```python
from build123d import *

# Parameters (mm, degrees)
SKETCH070_W         = 19.5
SKETCH070_H         = 35
PAD035_DEPTH        = 6
SKETCH074_W         = 15.5
SKETCH074_H         = 31
POCKET025_DEPTH     = 4
SKETCH071_W         = 11.5
SKETCH071_H         = 27
POCKET023_DEPTH     = 2.001
SKETCH069_W         = 11.5
SKETCH069_H         = 4
POCKET024_DEPTH     = 6.001
REVOLUTION007_ANGLE = 180
REVOLUTION008_ANGLE = -180


with BuildPart() as part:
    # Sketch070 → Pad035 (new body)
    with BuildSketch(Plane.XY):
        with Locations((9.75, 17.5)):
            Rectangle(SKETCH070_W, SKETCH070_H)
    extrude(amount=PAD035_DEPTH)

    # Sketch074 (on Face6 of Pad035) → Pocket025 (cut)
    with BuildSketch(Plane.XY.offset(6)):
        with Locations((9.75, 17.5)):
            Rectangle(SKETCH074_W, SKETCH074_H)
    extrude(amount=-POCKET025_DEPTH, mode=Mode.SUBTRACT)

    # Sketch071 (on Face11 of Pocket025) → Pocket023 (cut, through all)
    with BuildSketch(Plane.XY.offset(2)):
        with Locations((9.75, 17.5)):
            Rectangle(SKETCH071_W, SKETCH071_H)
    extrude(amount=-POCKET023_DEPTH, mode=Mode.SUBTRACT)

    # Sketch069 (on Face5 of Pocket023) → Pocket024 (cut, through all)
    with BuildSketch(Plane.XY.offset(6)):
        with Locations((9.75, 2)):
            Rectangle(SKETCH069_W, SKETCH069_H)
    extrude(amount=-POCKET024_DEPTH, mode=Mode.SUBTRACT)

    # Sketch075 (on Face18 of Pocket024) → Revolution007 (revolve)
    with BuildSketch(Plane.YZ.offset(2)):
        with BuildLine():
            ThreePointArc((6.5, 5), (5.5, 6), (4.5, 5))
            Line((4.5, 5), (6.5, 5))
        make_face()
        with BuildLine():
            ThreePointArc((30.5, 5), (29.5, 6), (28.5, 5))
            Line((28.5, 5), (30.5, 5))
        make_face()
    revolve(axis=Axis((2, 6.5, 5), (0, 1, 0)), revolution_arc=REVOLUTION007_ANGLE)

    # Sketch076 (on Face17 of Revolution007) → Revolution008 (revolve)
    with BuildSketch(Plane(origin=(17.5, 0, 0), x_dir=(0, -1, 0), z_dir=(-1, 0, 0))):
        with BuildLine():
            ThreePointArc((-28.5, 5), (-29.5, 6), (-30.5, 5))
            Line((-30.5, 5), (-28.5, 5))
        make_face()
        with BuildLine():
            ThreePointArc((-4.5, 5), (-5.5, 6), (-6.5, 5))
            Line((-6.5, 5), (-4.5, 5))
        make_face()
    revolve(axis=Axis((17.5, 6.5, 5), (0, 1, 0)), revolution_arc=REVOLUTION008_ANGLE)


solid = part.part
```
The model under review builds one solid part; all positions refer to its coordinate system, in mm. A direction names the side the tool comes from. Coordinates: 2 decimals unless noted, no trailing zeros. Write each loop counter-clockwise with the first axis right and the second up, starting at its lowest first coordinate (ties: lowest second). Pieces come first, ordered by that corner, then holes.
1) We need section C-C on x = 13. State the section outline as (y, z) points.
2) Machinability: for faces 1 (the face through (10, 33, 4)), 2 (the face through (15.5, 11.8, 1.7)), 3 (the face through (17, 0, 3)), which of the approach directions +Z, -Z, +X, -X, +Y, -Y give a long, thin tool a straight path to every point of the face, cutting with its end or side? Answer none if there is none.
3) We need section A-A on y = 25.5. State the section outline as (x, z) points, then the cut area to 3 significant figures.
4) We need section B-B on z = 5.6. State the section outline as (x, y) points, then the cut area to 3 significant figures.
5) To check wall thickness, follow probe 1 along X at (y, z) = (28, 3.95); probe 2 along X at (y, z) = (14, 1.5); probe 3 along Y at (x, z) = (11.75, 4.9). State the ranges of each line that lie inside material, in increasing order.
6) We need section D-D on z = 3.55. State the section outline as (x, y) points.
7) The part is to be moulded in two halves that separate along X. For faces 4 (the face through (16, 2, 4)), 5 (the face through (3, 18, 0)), 6 (the face through (19.5, 17, 3)), say which applies: pulls with the +X half, pulls with the -X half, needs draft (parallel to the pull), parting line crosses it, or undercut.
8) Clearance check with flat-ended pins moving along their axes: pin 1 Ø1.5 at (x, y) = (3.5, 29.5) entering from +Z; pin 2 Ø2 at (x, z) = (11, 0.5) entering from -Y; pin 3 Ø1.2 at (x, z) = (7, 4.5) entering from -Y. State where each tip first meets the part, or that it passes through.
Answer list:
1. outline: (31, 0) - (35, 0) - (35, 6) - (33, 6) - (33, 2) - (31, 2) - close
2. face 1: +Z
2. face 2: +Z, -Z, -Y
2. face 3: +Z, -Z, +X, -X, -Y
3. outline: (0, 0) - (4, 0) - (4, 2) - (2, 2) - (2, 6) - (0, 6) - close; (15.5, 0) - (19.5, 0) - (19.5, 6) - (17.5, 6) - (17.5, 2) - (15.5, 2) - close
3. area: 32.0 mm2
4. outline: (0, 0) - (4, 0) - (4, 2) - (2, 2) - (2, 4.7) arc R0.8 ccw to (2, 6.3) - (2, 28.7) arc R0.8 ccw to (2, 30.3) - (2, 33) - (17.5, 33) - (17.5, 30.3) arc R0.8 ccw to (17.5, 28.7) - (17.5, 6.3) arc R0.8 ccw to (17.5, 4.7) - (17.5, 2) - (15.5, 2) - (15.5, 0) - (19.5, 0) - (19.5, 35) - (0, 35) - close
4. area: 183 mm2
5. probe 1: x = 0 to 2, 17.5 to 19.5
5. probe 2: x = 0 to 4, 15.5 to 19.5
5. probe 3: y = 33 to 35
6. outline: (0, 0) - (4, 0) - (4, 2) - (2, 2) - (2, 33) - (17.5, 33) - (17.5, 2) - (15.5, 2) - (15.5, 0) - (19.5, 0) - (19.5, 35) - (0, 35) - close
7. face 4: undercut
7. face 5: needs draft
7. face 6: pulls with the +X half
8. pin 1: stops at z = 5.66
8. pin 2: stops at y = 31
8. pin 3: stops at y = 33
